Verification items for this drawing (mm, ordinates from the low corner). Coordinates: 2 decimals unless noted, no trailing zeros. Order: outer loops, then holes, each group sorted by start corner. A loop starts at its lowest first (then second) coordinate and runs counter-clockwise, first axis right, second up. Notation, with made-up numbers: (63, 39.25) -> (88, 39.25) arc R23 cw to (88, 66.25) -> close; hole circle Ø7 at (65.25, 7.25). An arc over 180 degrees is marked (long way). Write each question's results on one line, items separated by ' | '. Start each with the question number.
(1) Cross-section at B-B on x = 75. Enter the section's corners in (y, z), and give its area (3 significant figures).
(2) Cross-section at A-A on z = 47.5. Enter the section's corners in (x, y).
(3) Thickness scan on probe 1 along Z at (x, y) = (75, 5.5); probe 2 along Z at (x, y) = (68, 11) (1 decimal); probe 3 along X at (y, z) = (13.25, 66). Record the ranges inside material, lowest first. Write a range as [from, to].
(4) Draft check along X on the marked faces 1, 2 and 3. Enter one of: +X half, -X half, draft (parallel to the pull), parting line (faces both ways), or undercut.
(5) Cross-section at D-D on z = 77.5. Enter the section's corners in (x, y), and give its area (3 significant figures).
(6) Go/stop test with flat-tipped pins: pin 1 (1.5 mm diameter, centred on y = 11.5, z = 67, fed in from +X); pin 2 (4 mm diameter, centred on x = 19.5, y = 6.5, fed in from +Z) (1 decimal). Record where each tip stops, or that it passes through.
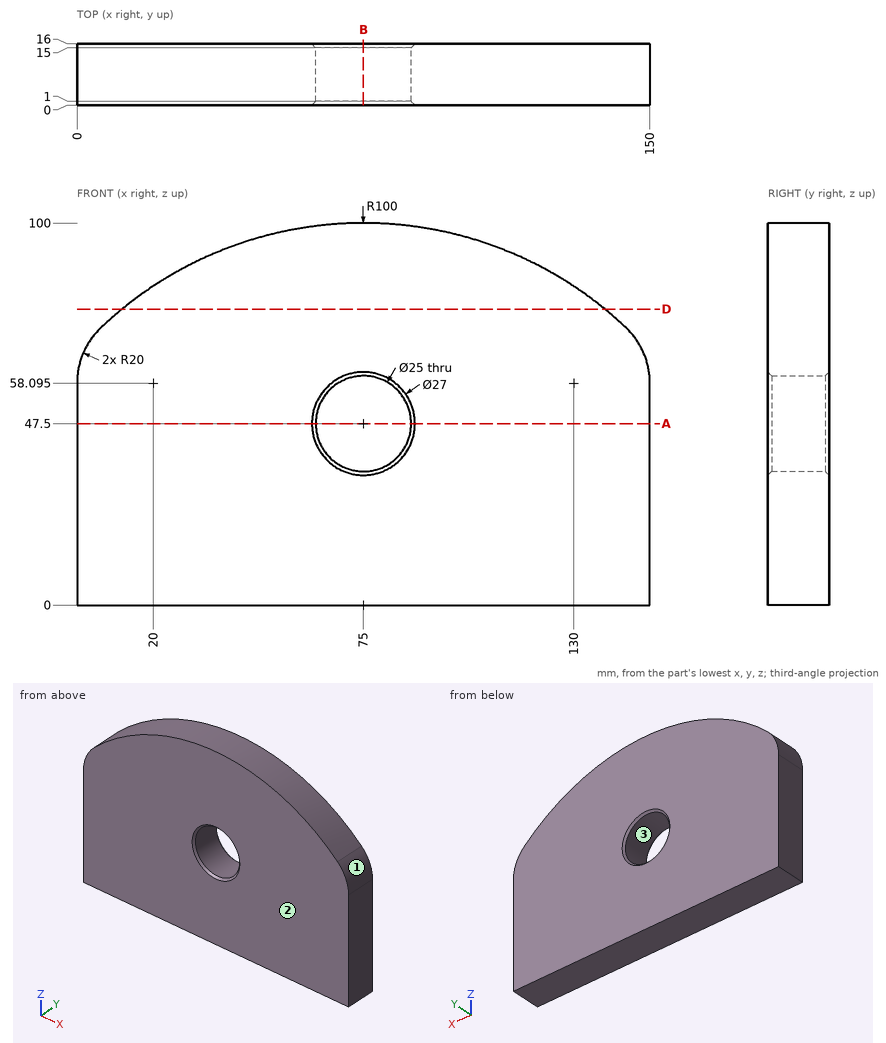
Results are:
1) outline: (0, 0) -> (16, 0) -> (16, 34) -> (15, 35) -> (1, 35) -> (0, 34) -> close; (0, 61) -> (1, 60) -> (15, 60) -> (16, 61) -> (16, 100) -> (0, 100) -> close | area: 1,200 mm2
2) outline: (0, 0) -> (61.5, 0) -> (62.5, 1) -> (62.5, 15) -> (61.5, 16) -> (0, 16) -> close; (87.5, 1) -> (88.5, 0) -> (150, 0) -> (150, 16) -> (88.5, 16) -> (87.5, 15) -> close
3) probe 1: z = [0, 35], [60, 100] | probe 2: z = [0, 37.1], [57.9, 99.8] | probe 3: x = [1.63, 148.37]
4) face 1: +X half | face 2: draft | face 3: undercut
5) outline: (11.8, 0) -> (138.2, 0) -> (138.2, 16) -> (11.8, 16) -> close | area: 2,020 mm2
6) pin 1: stops at x = 148.26 | pin 2: stops at z = 84.5
